Verification items for the finished model (mm, model axes). Face numbers are marked on the shaded views. A direction names the side the tool comes from. Round coordinates to 2 decimals unless told otherwise and drop trailing zeros. Order: outer loops, then holes, each group sorted by start corner. A loop starts at its lowest first (then second) coordinate and runs counter-clockwise, first axis right, second up. Notation, with made-up numbers: (-5.75, 65) -> (13.25, 65) arc R26 ccw to (13.25, 87) -> close; hole circle Ø2 at (38.25, 14.5). An arc over 180 degrees is marked (long way). Put each result on its own line as item: value.
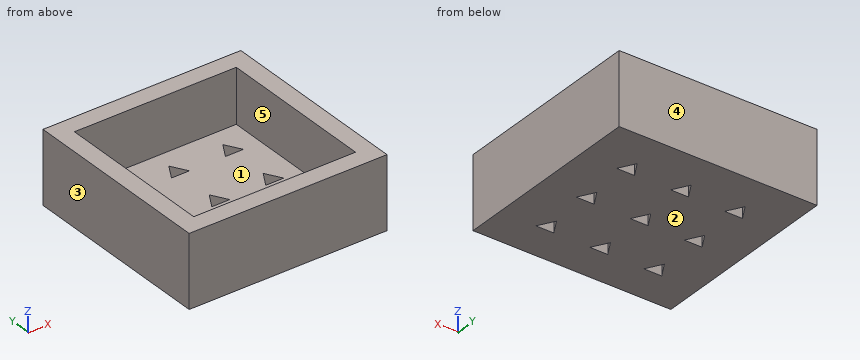
from build123d import *

# Parameters (mm, degrees)
F0_W     = 55
F0_H     = 54.330127
F1_DEPTH = 5
F2_W     = 55
F2_H     = 54.330127
F2_W_2   = 45
F2_H_2   = 44.330127
F3_DEPTH = 15


with BuildPart() as f1:
    # F0 (on Top) → F1 (new body)
    with BuildSketch(Plane.XY):
        with Locations((12.5, 17.165063)):
            Rectangle(F0_W, F0_H)
        Polygon((-5, 0), (-2.5, 4.330127), (0, 0), align=None, mode=Mode.SUBTRACT)
        Polygon((15, 0), (10, 0), (12.5, 4.330127), align=None, mode=Mode.SUBTRACT)
        Polygon((30, 0), (25, 0), (27.5, 4.330127), align=None, mode=Mode.SUBTRACT)
        Polygon((0, 15), (-5, 15), (-2.5, 19.330127), align=None, mode=Mode.SUBTRACT)
        Polygon((0, 30), (-5, 30), (-2.5, 34.330127), align=None, mode=Mode.SUBTRACT)
        Polygon((15, 15), (10, 15), (12.5, 19.330127), align=None, mode=Mode.SUBTRACT)
        Polygon((30, 15), (25, 15), (27.5, 19.330127), align=None, mode=Mode.SUBTRACT)
        Polygon((15, 30), (10, 30), (12.5, 34.330127), align=None, mode=Mode.SUBTRACT)
        Polygon((30, 30), (25, 30), (27.5, 34.330127), align=None, mode=Mode.SUBTRACT)
    extrude(amount=F1_DEPTH)

    # F2 (on face) → F3 (join)
    with BuildSketch(Plane.XY.offset(5)):
        with Locations((12.5, 17.165063)):
            Rectangle(F2_W, F2_H)
        with Locations((12.5, 17.165063)):
            Rectangle(F2_W_2, F2_H_2, mode=Mode.SUBTRACT)
    extrude(amount=F3_DEPTH)


solid = f1.part
Item 1: Material ranges on L1, parallel to Y at x = -3.5, z = 12.25; L2, parallel to X at y = 31.5, z = 7.75; L3, parallel to Z at x = 7.5, y = 13.5, recorded low to high. Write a range as [from, to].
Check sheet entries:
L1: y = [-10, -5], [39.33, 44.33]
L2: x = [-15, -10], [35, 40]
L3: z = [0, 5]
Item 2: Gauge pin test, flat end, axial feed: pin 1 Ø3 at (x, y) = (4, 30.5) entering from -Z. Record the tip position at first contact, or that the pin passes through.
Check sheet entries:
pin 1: stops at z = 0
Item 3: Section check B-B on y = 18. Record the boundary of the cut face in (x, z).
Check sheet entries:
outline: (-15, 0) -> (-3.27, 0) -> (-3.27, 5) -> (-10, 5) -> (-10, 20) -> (-15, 20) -> close; (-1.73, 0) -> (11.73, 0) -> (11.73, 5) -> (-1.73, 5) -> close; (13.27, 0) -> (26.73, 0) -> (26.73, 5) -> (13.27, 5) -> close; (28.27, 0) -> (40, 0) -> (40, 20) -> (35, 20) -> (35, 5) -> (28.27, 5) -> close
Item 4: Release check for a two-part mould opening along Y. For the marked faces 3, 4 and 5 record: +Y half, -Y half, draft (parallel to the pull), parting line (faces both ways), or undercut.
Check sheet entries:
face 3: draft
face 4: +Y half
face 5: undercut
Item 5: Section check C-C on y = 36.5. Record the boundary of the cut face in (x, z).
Check sheet entries:
outline: (-15, 0) -> (40, 0) -> (40, 20) -> (35, 20) -> (35, 5) -> (-10, 5) -> (-10, 20) -> (-15, 20) -> close
Item 6: Tool access check on the marked faces 1 and 2. Record the directions out of +Z, -Z, +X, -X, +Y, -Y that give a thin tool (end or side, any length) a straight path to the whole face; none if there is none.
Check sheet entries:
face 1: +Z
face 2: -Z, +X, -X, +Y, -Y
Item 7: Section check A-A on z = 13. Record the boundary of the cut face in (x, y).
Check sheet entries:
outline: (-15, -10) -> (40, -10) -> (40, 44.33) -> (-15, 44.33) -> close; hole (-10, -5) -> (35, -5) -> (35, 39.33) -> (-10, 39.33) -> close
Item 8: Section check D-D on z = 2. State how many separate pieces and enclosed holes the cut face has, then the cut area to 3 significant figures.
Check sheet entries:
separate pieces: 1
enclosed holes: 9
area: 2,890 mm^2
